For this review, use the dimensioned drawing (mm, ordinates from the lowest corner) and the shaded views. Coordinates: 2 decimals unless noted, no trailing zeros. Write each loop counter-clockwise with the first axis right and the second up, starting at its lowest first coordinate (ties: lowest second). Pieces come first, ordered by that corner, then holes. Notation, with made-up numbers: (80.5, -4) - (128.5, -4) arc R5 cw to (128.5, 0) - close; hole circle Ø7 at (15, 61). An arc over 180 degrees is marked (long way). Put each result on its own line as item: value.
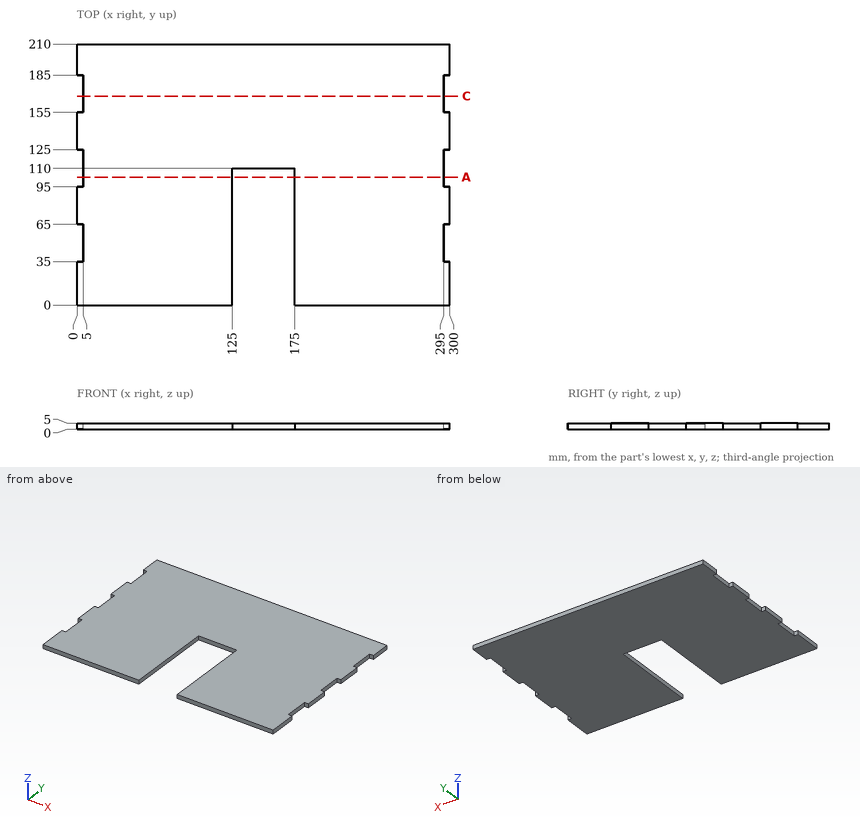
1. Consider section C-C on y = 168. State the section outline as (x, z) points.
Determined:
outline: (5, 0) - (295, 0) - (295, 5) - (5, 5) - close
2. For pin 1 Ø1.5 at (y, z) = (109, 4) entering from +X; pin 2 Ø2.5 at (y, z) = (116, 1.5) entering from -X, all flat-tipped, find the tip position at first contact; note any pin that passes through.
Determined:
pin 1: stops at x = 295
pin 2: stops at x = 5
3. To check wall thickness, follow probe 1 along X at (y, z) = (24.5, 4.6); probe 2 along X at (y, z) = (61.5, 1.3); probe 3 along Y at (x, z) = (138.5, 2.9). State the ranges of each line that lie inside material, in increasing order.
Determined:
probe 1: x = 0 to 125, 175 to 300
probe 2: x = 5 to 125, 175 to 295
probe 3: y = 110 to 210
4. Consider section A-A on y = 103. State the section outline as (x, z) points, plus the area to 3 significant figures.
Determined:
outline: (5, 0) - (125, 0) - (125, 5) - (5, 5) - close; (175, 0) - (295, 0) - (295, 5) - (175, 5) - close
area: 1,200 mm^2
